Work out the finished part from the listing and answer in its coordinate system (mm). A direction names the side the tool comes from. Give positions to 0.01 mm unless a question says otherwise; leave off trailing zeros. Order: outer loops, then holes, each group sorted by start corner. A loop starts at its lowest first (then second) coordinate and runs counter-clockwise, first axis right, second up. Notation, with made-up numbers: (30.5, -30.5) - (78.5, -30.5) arc R24 cw to (78.5, 8.5) - close; hole circle Ø3 at (7, 11). An arc over 180 degrees is marked (long way). Return JSON: item names as keys, results as strings. Group by question number.
from build123d import *

# Parameters (mm, degrees)
BOX003_W          = 28
BOX003_H          = 8
BOX003_DEPTH      = 10
CYLINDER_R        = 3.05
CYLINDER_DEPTH    = 80
CYLINDER001_R     = 3.05
CYLINDER001_DEPTH = 80
CYLINDER002_R     = 3.05
CYLINDER002_DEPTH = 80
BOX001_W          = 70
BOX001_H          = 24
BOX001_DEPTH      = 45
BOX002_W          = 80
BOX002_H          = 24
BOX002_DEPTH      = 43
BOX_W             = 147
BOX_H             = 24
BOX_DEPTH         = 51


with BuildPart() as slide_hole:
    # Box003 → Box003 (new body)
    with BuildSketch(Plane(origin=(18, 8, 0), x_dir=(1, 0, 0), z_dir=(0, 0, 1))):
        with Locations((14, 4)):
            Rectangle(BOX003_W, BOX003_H)
    extrude(amount=BOX003_DEPTH)


with BuildPart() as hole_r:
    # Cylinder → Cylinder (new body)
    with BuildSketch(Plane(origin=(136.95, 12, 0), x_dir=(1, 0, 0), z_dir=(0, 0, 1))):
        Circle(CYLINDER_R)
    extrude(amount=CYLINDER_DEPTH)


with BuildPart() as hole_c:
    # Cylinder001 → Cylinder001 (new body)
    with BuildSketch(Plane(origin=(111.95, 12, 0), x_dir=(1, 0, 0), z_dir=(0, 0, 1))):
        Circle(CYLINDER001_R)
    extrude(amount=CYLINDER001_DEPTH)


with BuildPart() as hole_l:
    # Cylinder002 → Cylinder002 (new body)
    with BuildSketch(Plane(origin=(86.95, 12, 0), x_dir=(1, 0, 0), z_dir=(0, 0, 1))):
        Circle(CYLINDER002_R)
    extrude(amount=CYLINDER002_DEPTH)


with BuildPart() as left_cut:
    # Box001 → Box001 (new body)
    with BuildSketch(Plane.XY.offset(6)):
        with Locations((35, 12)):
            Rectangle(BOX001_W, BOX001_H)
    extrude(amount=BOX001_DEPTH)


with BuildPart() as right_cut:
    # Box002 → Box002 (new body)
    with BuildSketch(Plane(origin=(78, 0, 0), x_dir=(1, 0, 0), z_dir=(0, 0, 1))):
        with Locations((40, 12)):
            Rectangle(BOX002_W, BOX002_H)
    extrude(amount=BOX002_DEPTH)


with BuildPart() as cut005:
    # Box → Box (new body)
    with BuildSketch(Plane.XY):
        with Locations((73.5, 12)):
            Rectangle(BOX_W, BOX_H)
    extrude(amount=BOX_DEPTH)

    # Cut: cut Right Cut
    add(right_cut.part, mode=Mode.SUBTRACT)

    # Cut001: cut Left Cut
    add(left_cut.part, mode=Mode.SUBTRACT)

    # Cut002: cut Hole L
    add(hole_l.part, mode=Mode.SUBTRACT)

    # Cut003: cut Hole C
    add(hole_c.part, mode=Mode.SUBTRACT)

    # Cut004: cut Hole R
    add(hole_r.part, mode=Mode.SUBTRACT)

    # Cut005: cut Slide Hole
    add(slide_hole.part, mode=Mode.SUBTRACT)


solid = cut005.part
1. The part is cut by section D-D (z = 23.5). Give the vertices of the cut face in (x, y), and give its area (3 significant figures).
2. Each of these flat-tipped pins is pushed along its axis until it touches: pin 1 (4 mm diameter, centred on y = 9.5, z = 25.5, fed in from +X); pin 2 (3 mm diameter, centred on y = 9.5, z = 35.5, fed in from -X); pin 3 (12 mm diameter, centred on x = 111, y = 10.5, fed in from -Z). Where does it stop, or does it pass through?
3. Consider probe 1 along X at (y, z) = (12, 48.25); probe 2 along Y at (x, z) = (86.95, 48.5); probe 3 along X at (y, z) = (7.75, 21). Determine where each line is inside the solid, lowest interval first. Write a range as from..to.
4. A tool of negligible diameter and unlimited length cuts with its end or side. For faces 1 (the flat face through (32, 8, 3)), 2 (the flat face through (70, 12, 28)), 3 (the flat face through (112, 18, 43)), from which of +Z, -Z, +X, -X, +Y, -Y can it reach the whole face along a straight path? Write none if from no direction.
5. The part is cut by section B-B (x = 136.95). Give the vertices of the cut face in (y, z), and give its area (3 significant figures).
6. The part is cut by section A-A (y = 12). Give the vertices of the cut face in (x, z).
7. Determine the mould class of faces 4 (the flat face through (46, 12, 3)), 5 (the flat face through (73, 24, 27)), 6 (the flat face through (78, 12, 21)) for opening direction Y: released by +Y, released by -Y, zero draft, split by the parting line, or undercut.
8. The part is cut by section C-C (x = 47.5). Give the vertices of the cut face in (y, z).
Answers:
{
 "1": {"outline": "(70, 0) - (78, 0) - (78, 24) - (70, 24) - close", "area": "192 mm^2"},
 "2": {"pin 1": "stops at x = 78", "pin 2": "stops at x = 70", "pin 3": "stops at z = 43"},
 "3": {"probe 1": "x = 70..83.9, 90..108.9, 115..133.9, 140..147", "probe 2": "y = 0..8.95, 15.05..24", "probe 3": "x = 70..78"},
 "4": {"face 1": "+Z, -Z", "face 2": "+Z, -X, +Y, -Y", "face 3": "-Z, +X, +Y, -Y"},
 "5": {"outline": "(0, 43) - (8.95, 43) - (8.95, 51) - (0, 51) - close; (15.05, 43) - (24, 43) - (24, 51) - (15.05, 51) - close", "area": "143 mm^2"},
 "6": {"outline": "(0, 0) - (18, 0) - (18, 6) - (0, 6) - close; (46, 0) - (78, 0) - (78, 43) - (83.9, 43) - (83.9, 51) - (70, 51) - (70, 6) - (46, 6) - close; (90, 43) - (108.9, 43) - (108.9, 51) - (90, 51) - close; (115, 43) - (133.9, 43) - (133.9, 51) - (115, 51) - close; (140, 43) - (147, 43) - (147, 51) - (140, 51) - close"},
 "7": {"face 4": "undercut", "face 5": "released by +Y", "face 6": "zero draft"},
 "8": {"outline": "(0, 0) - (24, 0) - (24, 6) - (0, 6) - close"}
}
